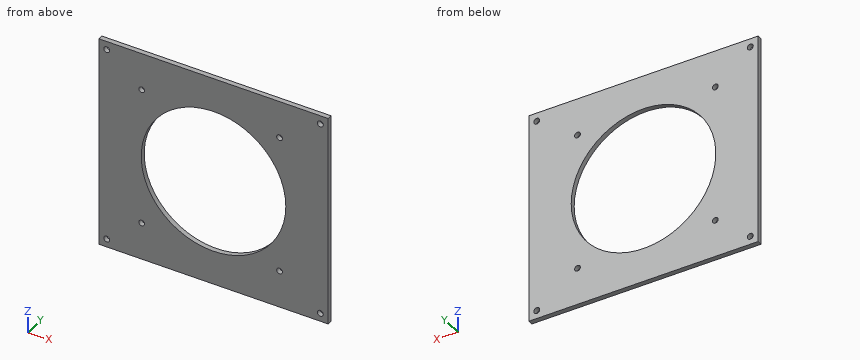
Autodesk Inventor part; units mm, degrees
ref_plane "Work Plane1" through (-59.5, 0, 0) normal (1, 0, 0) x (0, 0, -1)
ref_plane "YZ Plane" through (0, 0, 0) normal (1, 0, 0) x (0, 1, 0)
ref_plane "XZ Plane" through (0, 0, 0) normal (0, 1, 0) x (-1, 0, 0)
sketch "Sketch1" plane through (0, 0, 0) normal (0, 1, 0) x (-1, 0, 0)
  line L0 (0, 0) -> (119, 0)
  line L1 (119, 0) -> (119, -110.2)
  line L2 (119, -110.2) -> (0, -110.2)
  line L3 (0, -110.2) -> (0, 0)
  dimension "d0" = 119
  dimension "d1" = 110.2
extrude "Extrusion1" add sketch "Sketch1" along normal blind 2.5
sketch "Sketch2" plane through (0, 2.5, 0) normal (0, 1, 0) x (1, 0, 0)
  line L0 (-119, 0) -> (0, 0)
  line L1 (0, 0) -> (0, 110.2)
  line L2 (0, 110.2) -> (-119, 110.2)
  line L3 (-119, 110.2) -> (-119, 0)
  circle A0 centre (-114.875, 4.375) radius 1.55
  circle A1 centre (-11.5301, 10.067) radius 1.55
  circle A2 centre (-11.5301, 99.7072) radius 1.55
  circle A3 centre (-114.875, 105.95) radius 1.55
  dimension "d4" = 3.1
  dimension "d5" = 3.1
  dimension "d6" = 3.1
  dimension "d7" = 3.1
  dimension "d8" = 4.375
  dimension "d9" = 4.125
  dimension "d10" = 4.25
  dimension "d11" = 4.125
extrude "Extrusion2" cut sketch "Sketch2" against normal through all contours A0 | A3
ref_plane "Work Plane1" through (-59.5, 0, 0) normal (1, 0, 0) x (0, 0, -1)
mirror "Mirror1" about plane through (-59.5, 0, 0) normal (1, 0, 0) of "Extrusion2"
sketch "Sketch3" plane through (0, 2.5, 0) normal (0, 1, 0) x (1, 0, 0)
  circle A0 centre (-4.125, 4.375) radius 1.55
  circle A1 centre (-4.125, 105.95) radius 1.55
  circle A2 centre (-114.875, 4.375) radius 1.55
  circle A3 centre (-114.875, 105.95) radius 1.55
  line L0 (-119, 0) -> (0, 0)
  line L1 (0, 0) -> (0, 110.2)
  line L2 (0, 110.2) -> (-119, 110.2)
  line L3 (-119, 110.2) -> (-119, 0)
  circle A4 centre (-59.5, 55.1) radius 37.5
  circle A5 centre (-96.75, 90.85) radius 1.5
  circle A6 centre (-25.25, 90.85) radius 1.5
  circle A7 centre (-25.25, 19.35) radius 1.5
  circle A8 centre (-96.75, 19.35) radius 1.5
  dimension "d32" = 3
  dimension "d33" = 3
  dimension "d34" = 3
  dimension "d35" = 3
  dimension "d36" = 71.5
  dimension "d37" = 71.5
  dimension "d38" = 71.5
  dimension "d39" = 71.5
extrude "Extrusion3" cut sketch "Sketch3" against normal through all contours A4 | A5 | A6 | A7 | A8
properties part number "Base Cover Left 80mm fan"
Input: part model. Units: mm. Frame: model coordinates. Coordinates: 2 decimals unless noted, no trailing zeros. Order: outer loops, then holes, each group sorted by start corner. A loop starts at its lowest first (then second) coordinate and runs counter-clockwise, first axis right, second up. Notation, with made-up numbers: M 79,70.5 L 118,70.5 A17 ccw 118,79.5 Z; hole C 4.5,-0.75 d7. An arc over 180 degrees is marked long. Answer in a Markdown table with one row per item.
(1) Section query D-D, the plane y = 1.2. Give the number of separate pieces and of enclosed holes in the cut face, plus the area to 3 significant figures.
Numbers:
| item | result |
|---|---|
| separate pieces | 1 |
| enclosed holes | 9 |
| area | 8,640 mm^2 |
(2) Section query C-C, the plane z = -63.5. Output: boundary loops of the cut face in (x, y).
Numbers:
| item | result |
|---|---|
| outline | M -119,0 L -96.05,0 L -96.05,2.5 L -119,2.5 Z; M -22.95,0 L 0,0 L 0,2.5 L -22.95,2.5 Z |
(3) Section query A-A, the plane z = -105.95. Output: boundary loops of the cut face in (x, y) (3 decimals).
Numbers:
| item | result |
|---|---|
| outline | M -119,0 L -116.425,0 L -116.425,2.5 L -119,2.5 Z; M -113.325,0 L -5.675,0 L -5.675,2.5 L -113.325,2.5 Z; M -2.575,0 L 0,0 L 0,2.5 L -2.575,2.5 Z |
(4) Material intervals for line 1 (Z direction, x = -25.25, y = 1.9); line 2 (Z direction, x = -59.5, y = 1); line 3 (X direction, y = 1.95, z = -55.1), sorted ascending. Write a range as [from, to].
Numbers:
| item | result |
|---|---|
| line 1 | z = [-110.2, -92.35], [-89.35, -70.37], [-39.83, -20.85], [-17.85, 0] |
| line 2 | z = [-110.2, -92.6], [-17.6, 0] |
| line 3 | x = [-119, -97], [-22, 0] |
(5) Section query B-B, the plane x = -59.5. Output: boundary loops of the cut face in (y, z), plus the area to 3 significant figures.
Numbers:
| item | result |
|---|---|
| outline | M 0,-110.2 L 2.5,-110.2 L 2.5,-92.6 L 0,-92.6 Z; M 0,-17.6 L 2.5,-17.6 L 2.5,0 L 0,0 Z |
| area | 88.0 mm^2 |
